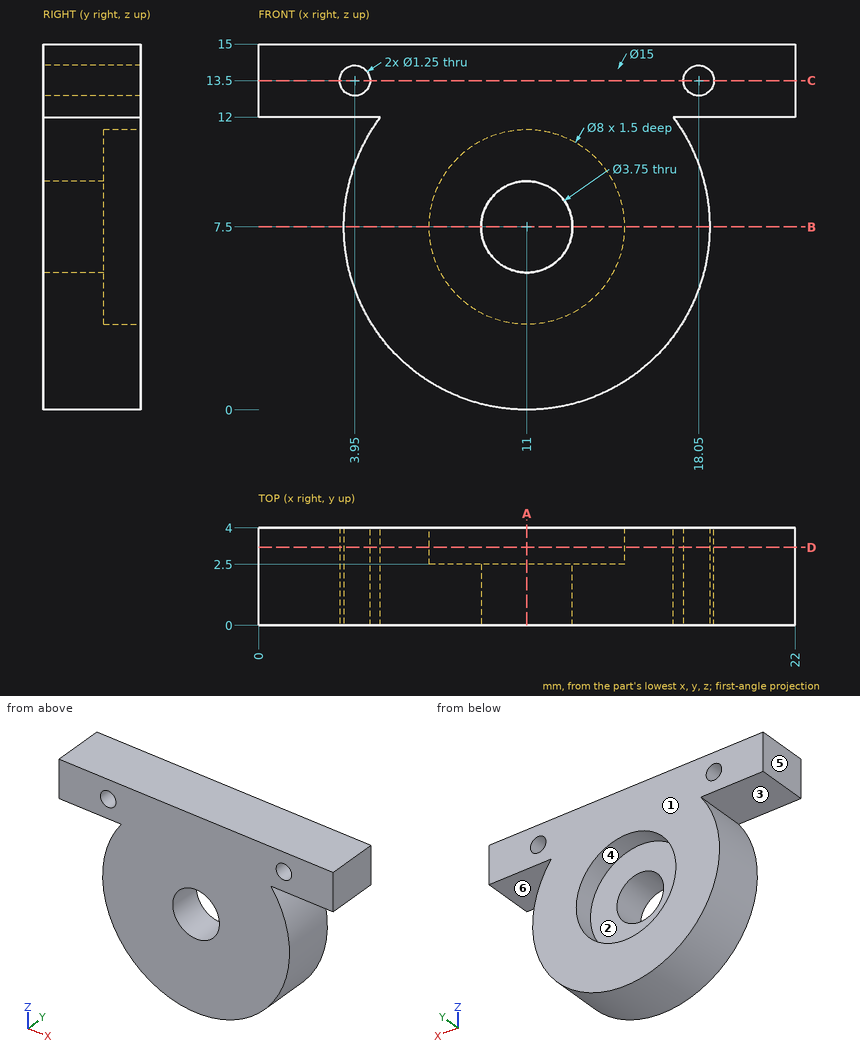
Study the drawing (mm; zero at the part's minimum x, y, z) and answer. A direction names the side the tool comes from. Round coordinates to 2 decimals unless told otherwise and drop trailing zeros. Write each loop counter-clockwise with the first axis right and the second up, starting at its lowest first coordinate (ties: lowest second). Pieces come first, ordered by that corner, then holes.
Q1. Find section A-A on x = 11. Determine the outline of the cut face in (y, z) (3 decimals), and give its area (3 significant figures).
Values:
outline: (0, 0) - (4, 0) - (4, 3.5) - (2.5, 3.5) - (2.5, 5.625) - (0, 5.625) - close; (0, 9.375) - (2.5, 9.375) - (2.5, 11.5) - (4, 11.5) - (4, 15) - (0, 15) - close
area: 38.6 mm2
Q2. Find section B-B on z = 7.5. Determine the outline of the cut face in (x, y) (3 decimals), and give its area (3 significant figures).
Values:
outline: (3.5, 0) - (9.125, 0) - (9.125, 2.5) - (7, 2.5) - (7, 4) - (3.5, 4) - close; (12.875, 0) - (18.5, 0) - (18.5, 4) - (15, 4) - (15, 2.5) - (12.875, 2.5) - close
area: 38.6 mm2
Q3. A flat-ended cylindrical pin translates along its axis: P1, Ø2, axis at x = 18.5, y = 2.5, coming from the -Z side. Find the tip coordinate at first contact, or state that the pin passes through.
Values:
P1: stops at z = 3.76
Q4. Straight lines are drawn through the part: line 1 (X direction, y = 1.75, z = 13.5) (3 decimals); line 2 (X direction, y = 3.2, z = 7.5); line 3 (Y direction, x = 11.25, z = 10). For each, find the intervals that lie inside material, in ascending order.
Values:
line 1: x = 0 to 3.325, 4.575 to 17.425, 18.675 to 22
line 2: x = 3.5 to 7, 15 to 18.5
line 3: y = 0 to 2.5
Q5. Find section C-C on z = 13.5. Determine the outline of the cut face in (x, y) (3 decimals), and give its area (3 significant figures).
Values:
outline: (0, 0) - (3.325, 0) - (3.325, 4) - (0, 4) - close; (4.575, 0) - (17.425, 0) - (17.425, 4) - (4.575, 4) - close; (18.675, 0) - (22, 0) - (22, 4) - (18.675, 4) - close
area: 78.0 mm2
Q6. Find section D-D on y = 3.2. Determine the outline of the cut face in (x, z) (3 decimals), and give its area (3 significant figures).
Values:
outline: (0, 12) - (5, 12) arc R7.5 ccw (long way) to (17, 12) - (22, 12) - (22, 15) - (0, 15) - close; hole circle Ø1.25 at (3.95, 13.5); hole circle Ø8 at (11, 7.5); hole circle Ø1.25 at (18.05, 13.5)
area: 165 mm2
Q7. The mould has two halves that part along X. Classify the marked faces 4, 5 and 6: released by +X, released by -X, zero draft, split by the parting line, or undercut.
Values:
face 4: undercut
face 5: released by -X
face 6: zero draft
Q8. A tool of negligible diameter and unlimited length cuts with its end or side. For the marked faces 1, 2 and 3, from which of +Z, -Z, +X, -X, +Y, -Y can it reach the whole face along a straight path? Write none if from no direction.
Values:
face 1: +Z, -Z, +X, -X, +Y
face 2: +Y
face 3: -X, +Y, -Y
